from build123d import *

# Parameters (mm, degrees)
F1_DEPTH = 5


with BuildPart() as f1:
    # F0 (on Top) → F1 (new body)
    with BuildSketch(Plane.XY):
        with BuildLine():
            Line((-54.998, -10), (0, -10))
            Line((0, -10), (0, 0))
            Line((0, 0), (-80, 0))
            Line((-80, 0), (-80, -13))
            Line((-80, -13), (-60, -13))
            ThreePointArc((-60, -13), (-57.914334, -10.807501), (-54.998, -10))
        make_face()
        with BuildLine():
            ThreePointArc((54.998, -10), (57.914334, -10.807501), (60, -13))
            Line((60, -13), (80, -13))
            Line((80, -13), (80, 0))
            Line((80, 0), (0, 0))
            Line((0, 0), (0, -10))
            Line((0, -10), (54.998, -10))
        make_face()
        with BuildLine():
            Line((-80, 0), (0, 0))
            Line((0, 0), (0, 10))
            Line((0, 10), (-54.998, 10))
            ThreePointArc((-54.998, 10), (-57.914334, 10.807501), (-60, 13))
            Line((-60, 13), (-80, 13))
            Line((-80, 13), (-80, 0))
        make_face()
        with BuildLine():
            Line((0, 0), (80, 0))
            Line((80, 0), (80, 13))
            Line((80, 13), (60, 13))
            ThreePointArc((60, 13), (57.916618, 10.80758), (55.002, 10))
            Line((55.002, 10), (0, 10))
            Line((0, 10), (0, 0))
        make_face()
    extrude(amount=F1_DEPTH)


solid = f1.part
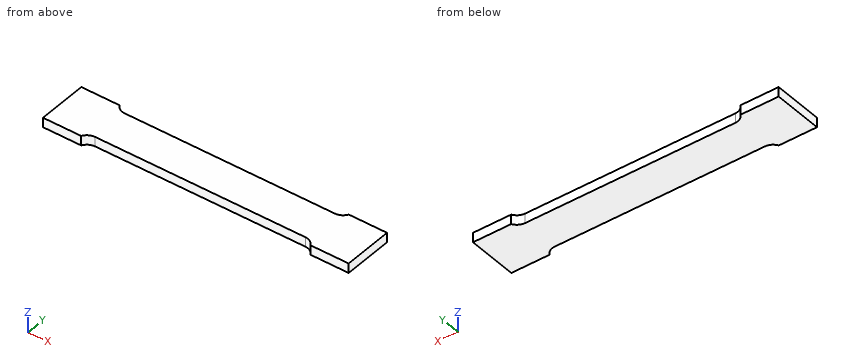
Verification items for the finished model (mm, model axes). Give positions to 0.01 mm unless a question says otherwise; leave off trailing zeros. Loops run counter-clockwise (first coordinate to the right, second up) from the corner with the lowest first, then second, coordinate; pieces in that order, holes last. Notation, with made-up numbers: (-26.75, 1.25) - (12.25, 1.25) arc R29 cw to (12.25, 30.25) - close; hole circle Ø7 at (-40, 40.5). An arc over 180 degrees is marked (long way). Write each question's results on one line, items separated by ' | '.
1) Sectioned sample at C-C on x = 31. Record the boundary of the cut face in (y, z), plus the area to 3 significant figures.
Solution:
outline: (-10, 0) - (10, 0) - (10, 5) - (-10, 5) - close | area: 100 mm2
2) Sectioned sample at B-B on z = 3.25. Record the boundary of the cut face in (x, y), plus the area to 3 significant figures.
Solution:
outline: (-80, -13) - (-60, -13) arc R5.67 cw to (-55, -10) - (55, -10) arc R5.67 cw to (60, -13) - (80, -13) - (80, 13) - (60, 13) arc R5.66 cw to (55, 10) - (-55, 10) arc R5.67 cw to (-60, 13) - (-80, 13) - close | area: 3,460 mm2
3) Material ranges on L1, parallel to Y at x = 21, z = 1.5; L2, parallel to X at y = -12, z = 4.7; L3, parallel to Y at x = -59.5, z = 0.7, recorded low to high. Write a range as from..to.
Solution:
L1: -10..10 | L2: -80..-59.32, 59.32..80 | L3: -12.22..12.22
4) Sectioned sample at A-A on y = -11.5. Record the boundary of the cut face in (x, z).
Solution:
outline: (-80, 0) - (-58.84, 0) - (-58.84, 5) - (-80, 5) - close; (58.84, 0) - (80, 0) - (80, 5) - (58.84, 5) - close
